Autodesk Inventor part; units mm, degrees
ref_plane "Work Plane1" through (29, 0, 0) normal (0, -1, 0) x (1, 0, 0)
ref_plane "YZ Plane" through (0, 0, 0) normal (1, 0, 0) x (0, 1, 0)
ref_plane "XZ Plane" through (0, 0, 0) normal (0, 1, 0) x (-1, 0, 0)
sketch "Sketch1" plane through (0, 0, 0) normal (0, 0, 1) x (1, 0, 0)
  line L0 (0.1778, 0) -> (15.875, 0)
  line L1 (15.875, 0) -> (15.875, 3.175)
  line L2 (15.875, 3.175) -> (2.5402, 3.175)
  line L3 (2.5402, 3.175) -> (0.0001, 3.175)
  line L4 (0.0001, 3.175) -> (0, 3.175)
  line L5 (0, 3.175) -> (0, 5.5499)
  line L6 (0, 5.5499) -> (-3.3528, 5.5499)
  line L7 (-3.3528, 5.5499) -> (-3.3528, 2.2877)
  line L8 (-3.3528, 2.2877) -> (-1.143, 2.2877)
  line L9 (-1.143, 2.2877) -> (0.1778, 0)
  line L10 (-7.1984, 0) -> (19.7206, 0)
  line L11 (0, -1.11) -> (0, 6.6599)
  line L12 (2.5402, 3.175) -> (0, 3.175) construction
  dimension "d1" = 13.3348
  dimension "d2" = 2.5401
  dimension "d3" = 3.3528
  dimension "d4" = 2.2098
  dimension "d5" = 60
  dimension "d6" = 6.35
  dimension "d7" = 6.35
  dimension "d8" = 4.5754
  dimension "d9" = 11.0998
  dimension "d26" = 15.875
revolve "Body" add sketch "Sketch1" angle 360 about axis through (0.1778, 0, 0) along (1, 0, 0) contours L9 L11 L3 L2 L1 L0 | L9 L8 L7 L6 L5 L11
sketch "Sketch2" plane through (-3.3528, 0, 0) normal (-1, 0, 0) x (0, 0, 1)
  circle A0 centre (0, 0) radius 2.2877
  line L0 (0, -7.7699) -> (0, 7.7699)
  line L1 (-7.7699, 0) -> (7.7699, 0)
  line L2 (2.2877, 0) -> (1.1438, -1.9812)
  line L3 (1.1438, -1.9812) -> (-1.1438, -1.9812)
  line L4 (-1.1438, -1.9812) -> (-2.2877, 0)
  line L5 (-2.2877, 0) -> (-1.1438, 1.9812)
  line L6 (-1.1438, 1.9812) -> (1.1438, 1.9812)
  line L7 (1.1438, 1.9812) -> (2.2877, 0)
  point P0 (0, 0)
extrude "Slot" add sketch "Sketch2" against normal up to next contours L7 A0 | A0 L2 | L6 L0 A0 | A0 L0 L3 | L0 L6 A0 | A0 L3 L0 | L4 A0 | A0 L5
fillet "Fillet1" radius 2.9718 1 edges at (-3.3528, -5.5499, 0)
thread "Thread"
chamfer "Chamfer1" distance 0.779 distance2 0.779 1 edges at (15.875, -3.175, 0) measured on face at (15.875, 0.0983, -0.8099)
ref_plane "Work Plane1" through (29, 0, 0) normal (0, -1, 0) x (1, 0, 0)
fillet "Fillet2" radius 0.1 1 edges at (0.0001, -3.175, 0)
equation "\"d1\" = GEL"
equation "\"d3\" = KOH"
equation "\"d4\" = INTI"
equation "\"d6\" = GD"
equation "\"d7\" = BDM"
equation "\"d8\" = 1.1547 * SW"
equation "\"d9\" = KOD"
equation "\"d26\" = NLG"
equation "\"d30\" = R"
equation "\"d17\" = RR"
equation "\"d13\" = GEL"
equation "\"d15\" = -0.5 * SPD + 0.5 * GD"
equation "\"d16\" = GUL"
equation "\"GD\" = NND"
equation "\"NLG\" = 15.875"
equation "\"GEL\" = 13.3348"
equation "\"KOD\" = 11.0998"
equation "\"KOH\" = 3.3528"
equation "\"INTI\" = 2.2098"
equation "\"GAL\" = 2.54"
equation "\"GUL\" = 0.77902"
equation "\"BDM\" = NND"
equation "\"SW\" = 3.9624"
equation "\"RR\" = 2.9718"
equation "\"SPD\" = 4.79196"
equation "\"R\" = 0.1"
equation "\"TOA\" = 30deg"
equation "\"GD1\" = SPD"
equation "\"THREADDIA\" = 6.35"
equation "\"KOH1\" = 0.7874"
equation "\"NND\" = 6.35"
equation "\"E0\" = 4.57657"
properties part number "ANSI B18.3 - 1/4 - 20 x 5/8" material "Steel, Mild"
The listing builds one solid part. Answer for the finished solid, in the listing's coordinates (mm). A direction names the side the tool comes from. Round coordinates to 2 decimals unless told otherwise and drop trailing zeros. Order: outer loops, then holes, each group sorted by start corner. A loop starts at its lowest first (then second) coordinate and runs counter-clockwise, first axis right, second up. Notation, with made-up numbers: (46.25, 63.25) -> (61.25, 63.25) arc R20 cw to (61.25, 86.25) -> close; hole circle Ø1 at (45.5, 77.5). An arc over 180 degrees is marked (long way). Put each result on its own line as item: value.
Q1. Which of the six approach directions +Z, -Z, +X, -X, +Y, -Y give full straight-line access (tool end or side, diameter ignored) to faces 4 (the flat face through (-2.18, 1, 1.71)), 5 (the flat face through (-3.353, 1, 2)), 6 (the cylindrical face through (7.49, -0.69, 3.1))?
Results list:
face 4: -X
face 5: +Z, -Z, -X, +Y, -Y
face 6: +X
Q2. Consider line 1 along Z through (x, y) = (-1.5, 0.75); line 2 along Y through (x, z) = (-2, -0.5); line 3 along Y through (x, z) = (8.5, 1.5). Determine where each line is inside the solid, lowest interval first.
Results list:
line 1: -5.28 to -1.85, 1.85 to 5.28
line 2: -5.05 to -1.98, 1.98 to 5.05
line 3: -2.8 to 2.8
Q3. Each of these flat-tipped pins is pushed along its axis until it touches: P1, Ø3, axis at y = -1, z = -0.5, coming from the -X side; P2, Ø4, axis at x = 9, z = -3.5, coming from the +Y side; P3, Ø5, axis at x = 9.5, z = 0.5, coming from the +Y side (3 decimals); P4, Ø1, axis at y = -1.5, z = -3, coming from the -X side. Where does it stop, or does it pass through?
Results list:
P1: x = -3.35
P2: y = 2.8
P3: y = 3.175
P4: x = -3.34
Q4. Section A-A, the plane x = 12.75 is taken. Write down the section's boundary in (y, z) (3 decimals).
Results list:
outline: circle Ø6.35 at (0, 0)
Q5. Determine the mould class of faces 1 (the cylindrical face through (-0.193, 5.127, 2.126)), 2 (the flat face through (15.875, 0, 0)), 3 (the flat face through (-2.18, 0.98, -1.72)) for opening direction Y: pulls with the +Y half, pulls with the -Y half, needs draft (parallel to the pull), parting line crosses it, or undercut.
Results list:
face 1: parting line crosses it
face 2: needs draft
face 3: undercut
